Design review of the part built by this model. Coordinates are the model's own, in mm. Coordinates: 2 decimals unless noted, no trailing zeros. Write item = value, one per line. Start each with the question number.
```python
from build123d import *

# Parameters (mm, degrees)
BOSS_EXTRUDE1_DEPTH = 1.5748
SKETCH2_R           = 1.5
SKETCH2_R_2         = 0.3
SKETCH2_R_3         = 0.508
SKETCH2_R_4         = 0.5969
SKETCH2_R_5         = 0.449999989
SKETCH2_R_6         = 0.4064
SKETCH2_R_7         = 0.9017
SKETCH2_R_8         = 0.350000062
CUT_EXTRUDE1_DEPTH  = 2.5748


with BuildPart() as part:
    # Sketch1 → Boss-Extrude1 (new body)
    with BuildSketch(Plane(origin=(0, 0, 0), x_dir=(1, 0, 0), z_dir=(0, 1, 0))):
        with BuildLine():
            Line((-28.575, 26.67), (28.575, 26.67))
            ThreePointArc((28.575, 26.67), (30.371051224, 25.926051224), (31.115, 24.13))
            Line((31.115, 24.13), (31.115, -24.13))
            ThreePointArc((31.115, -24.13), (30.371051224, -25.926051224), (28.575, -26.67))
            Line((28.575, -26.67), (-28.575, -26.67))
            ThreePointArc((-28.575, -26.67), (-30.371051224, -25.926051224), (-31.115, -24.13))
            Line((-31.115, -24.13), (-31.115, 24.13))
            ThreePointArc((-31.115, 24.13), (-30.371051224, 25.926051224), (-28.575, 26.67))
        make_face()
    extrude(amount=BOSS_EXTRUDE1_DEPTH)

    # Sketch2 → Cut-Extrude1 (cut, through all)
    with BuildSketch(Plane(origin=(0, 1.5748, 0), x_dir=(1, 0, 0), z_dir=(0, 1, 0))):
        with Locations((-28.575, 24.13)):
            Circle(SKETCH2_R)
        with Locations((28.575, 24.13)):
            Circle(SKETCH2_R)
        with Locations((28.575, -24.13)):
            Circle(SKETCH2_R)
        with Locations((-28.575, -24.13)):
            Circle(SKETCH2_R)
        with Locations((-20.955, 17.78)):
            Circle(SKETCH2_R_2)
        with Locations((14.605, 20.32)):
            Circle(SKETCH2_R_3)
        with Locations((12.065, 20.32)):
            Circle(SKETCH2_R_3)
        with Locations((9.525, 20.32)):
            Circle(SKETCH2_R_3)
        with Locations((6.985, 20.32)):
            Circle(SKETCH2_R_3)
        with Locations((4.445, 20.32)):
            Circle(SKETCH2_R_3)
        with Locations((1.905, 20.32)):
            Circle(SKETCH2_R_3)
        with Locations((-0.635, 20.32)):
            Circle(SKETCH2_R_3)
        with Locations((-3.175, 20.32)):
            Circle(SKETCH2_R_3)
        with Locations((-5.715, 20.32)):
            Circle(SKETCH2_R_3)
        with Locations((-8.255, 20.32)):
            Circle(SKETCH2_R_3)
        with Locations((-10.795, 20.32)):
            Circle(SKETCH2_R_3)
        with Locations((-13.335, 20.32)):
            Circle(SKETCH2_R_3)
        with Locations((-15.875, 20.32)):
            Circle(SKETCH2_R_3)
        with Locations((12.065, 17.78)):
            Circle(SKETCH2_R_3)
        with Locations((9.525, 17.78)):
            Circle(SKETCH2_R_3)
        with Locations((6.985, 17.78)):
            Circle(SKETCH2_R_3)
        with Locations((4.445, 17.78)):
            Circle(SKETCH2_R_3)
        with Locations((1.905, 17.78)):
            Circle(SKETCH2_R_3)
        with Locations((-0.635, 17.78)):
            Circle(SKETCH2_R_3)
        with Locations((-3.175, 17.78)):
            Circle(SKETCH2_R_3)
        with Locations((-5.715, 17.78)):
            Circle(SKETCH2_R_3)
        with Locations((-8.255, 17.78)):
            Circle(SKETCH2_R_3)
        with Locations((-10.795, 17.78)):
            Circle(SKETCH2_R_3)
        with Locations((-13.335, 17.78)):
            Circle(SKETCH2_R_3)
        with Locations((-15.875, 17.78)):
            Circle(SKETCH2_R_3)
        with Locations((14.605, 17.78)):
            Circle(SKETCH2_R_3)
        with Locations((4.445, 13.97)):
            Circle(SKETCH2_R_2)
        with Locations((-24.6634, -11.4808)):
            Circle(SKETCH2_R_4)
        with Locations((-24.6634, -16.4592)):
            Circle(SKETCH2_R_4)
        with Locations((-12.1666, -16.4592)):
            Circle(SKETCH2_R_4)
        with Locations((-12.1666, -11.4808)):
            Circle(SKETCH2_R_4)
        with Locations((-23.495, -22.86)):
            Circle(SKETCH2_R_5)
        with Locations((-13.335, -22.86)):
            Circle(SKETCH2_R_5)
        with Locations((-6.985, -13.97)):
            Circle(SKETCH2_R_6)
        with Locations((-4.445, -13.97)):
            Circle(SKETCH2_R_6)
        with Locations((-18.415, -9.4742)):
            Circle(SKETCH2_R_7)
        with Locations((-18.415, -18.47)):
            Circle(SKETCH2_R_7)
        with Locations((7.0866, -11.4808)):
            Circle(SKETCH2_R_4)
        with Locations((7.0866, -16.4592)):
            Circle(SKETCH2_R_4)
        with Locations((19.5834, -16.4592)):
            Circle(SKETCH2_R_4)
        with Locations((19.5834, -11.4808)):
            Circle(SKETCH2_R_4)
        with Locations((24.765, -13.97)):
            Circle(SKETCH2_R_6)
        with Locations((27.305, -13.97)):
            Circle(SKETCH2_R_6)
        with Locations((13.335, -9.4742)):
            Circle(SKETCH2_R_7)
        with Locations((13.335, -18.47)):
            Circle(SKETCH2_R_7)
        with Locations((7.0866, 8.8392)):
            Circle(SKETCH2_R_4)
        with Locations((7.0866, 3.8608)):
            Circle(SKETCH2_R_4)
        with Locations((19.5834, 3.8608)):
            Circle(SKETCH2_R_4)
        with Locations((19.5834, 8.8392)):
            Circle(SKETCH2_R_4)
        with Locations((24.765, 6.35)):
            Circle(SKETCH2_R_6)
        with Locations((27.305, 6.35)):
            Circle(SKETCH2_R_6)
        with Locations((13.335, 10.8458)):
            Circle(SKETCH2_R_7)
        with Locations((13.335, 1.85)):
            Circle(SKETCH2_R_7)
        with Locations((-24.6634, 8.8392)):
            Circle(SKETCH2_R_4)
        with Locations((-24.6634, 3.8608)):
            Circle(SKETCH2_R_4)
        with Locations((-12.1666, 3.8608)):
            Circle(SKETCH2_R_4)
        with Locations((-12.1666, 8.8392)):
            Circle(SKETCH2_R_4)
        with Locations((-6.985, 6.35)):
            Circle(SKETCH2_R_6)
        with Locations((-4.445, 6.35)):
            Circle(SKETCH2_R_6)
        with Locations((-18.415, 10.8458)):
            Circle(SKETCH2_R_7)
        with Locations((-18.415, 1.85)):
            Circle(SKETCH2_R_7)
        with Locations((8.255, -22.86)):
            Circle(SKETCH2_R_5)
        with Locations((18.415, -22.86)):
            Circle(SKETCH2_R_5)
        with Locations((8.255, -3.81)):
            Circle(SKETCH2_R_5)
        with Locations((18.415, -3.81)):
            Circle(SKETCH2_R_5)
        with Locations((-23.495, -3.81)):
            Circle(SKETCH2_R_5)
        with Locations((-13.335, -3.81)):
            Circle(SKETCH2_R_5)
        with Locations((-6.985, -8.89)):
            Circle(SKETCH2_R_8)
    extrude(amount=-CUT_EXTRUDE1_DEPTH, mode=Mode.SUBTRACT)


solid = part.part
```
(1) For pin 1 Ø1.4 at (x, z) = (-18.415, 18.47) entering from +Y, flat-tipped, find the tip position at first contact; note if it passes through.
(2) Take a section at A-A, the plane y = 0.5. Count the separate pieces of the cut face and the enclosed holes in it, then the cut area to 3 significant figures.
(3) For line 1 (X direction, y = 0.8, z = 16.5) (3 decimals); line 2 (X direction, y = 1.3, z = -23) (3 decimals); line 3 (X direction, y = 0.5, z = 16) (3 decimals), list the stretches that pass through material, from the lowest coordinate up.
(4) Mouldability with a two-part tool opening along Z and no side actions: class faces 1 (the face through (-19.13, 0.8, 19.02)), 2 (the face through (31.115, 1, 0)), 3 (the face through (30.351, 0.776, -25.946)) as pulls with the +Z half, pulls with the -Z half, needs draft (parallel to the pull), parting line crosses it, or undercut.
Report:
q1.pin_1 = through
q2.separate_pieces = 1
q2.enclosed_holes = 73
q2.area = 3,220 mm2
q3.line_1 = -31.115 to -25.259, -24.068 to -12.762, -11.571 to 6.491, 7.682 to 18.988, 20.179 to 31.115
q3.line_2 = -31.115 to -29.561, -27.589 to 27.589, 29.561 to 31.115
q3.line_3 = -31.115 to -25.045, -24.282 to -12.548, -11.785 to 6.705, 7.468 to 19.202, 19.965 to 31.115
q4.face_1 = undercut
q4.face_2 = needs draft
q4.face_3 = pulls with the -Z half
